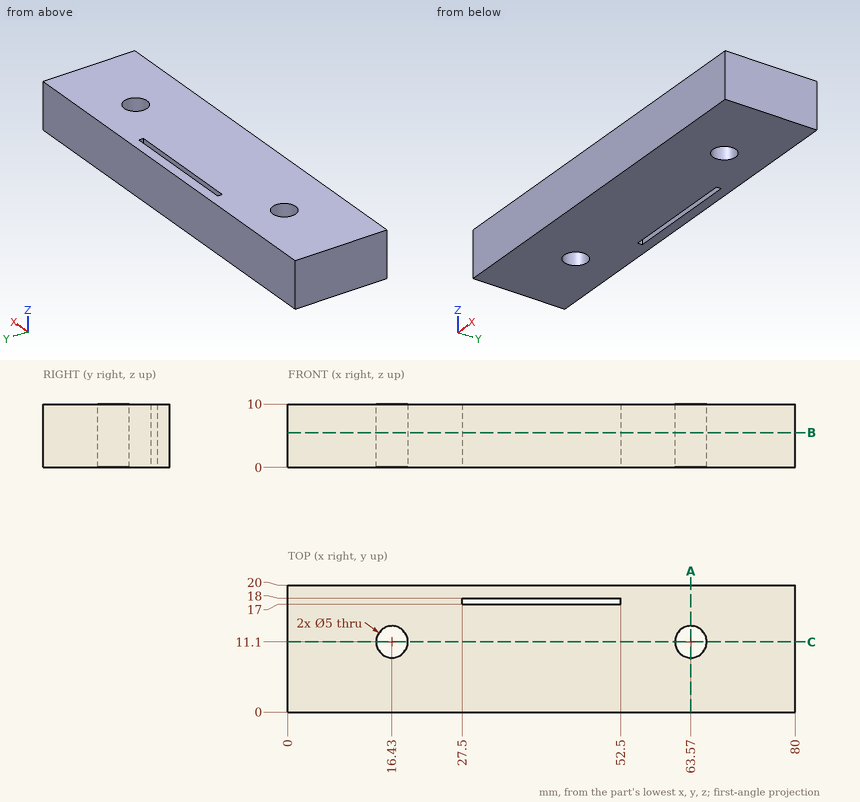
Source: three-view drawing plus pictorial views. Frame: mm from the lowest corner of the part. Give positions to 0.01 mm unless a question says otherwise; leave off trailing zeros. Order: outer loops, then holes, each group sorted by start corner. A loop starts at its lowest first (then second) coordinate and runs counter-clockwise, first axis right, second up. Notation, with made-up numbers: (-21, -11.5) -> (-8, -11.5) arc R27 ccw to (-8, 25.5) -> close; hole circle Ø8 at (11.25, 62). An arc over 180 degrees is marked (long way). Put each result on its own line as item: value.
Q1. Material intervals for L1, parallel to X at y = 11.25, z = 0.75; L2, parallel to Y at x = 63.57, z = 2.75; L3, parallel to X at y = 10, z = 8 (3 decimals), sorted ascending.
Here are the results:
L1: x = 0 to 13.93, 18.93 to 61.07, 66.07 to 80
L2: y = 0 to 8.6, 13.6 to 20
L3: x = 0 to 14.185, 18.675 to 61.325, 65.815 to 80
Q2. Section C-C, the plane y = 11.1. Return loops of the section in (x, z), then the cut area to 3 significant figures.
Here are the results:
outline: (0, 0) -> (13.93, 0) -> (13.93, 10) -> (0, 10) -> close; (18.93, 0) -> (61.07, 0) -> (61.07, 10) -> (18.93, 10) -> close; (66.07, 0) -> (80, 0) -> (80, 10) -> (66.07, 10) -> close
area: 700 mm^2
Q3. Section B-B, the plane z = 5.5. Return loops of the section in (x, y).
Here are the results:
outline: (0, 0) -> (80, 0) -> (80, 20) -> (0, 20) -> close; hole circle Ø5 at (16.43, 11.1); hole (27.5, 17) -> (52.5, 17) -> (52.5, 18) -> (27.5, 18) -> close; hole circle Ø5 at (63.57, 11.1)
Q4. Section A-A, the plane x = 63.57. Return loops of the section in (y, z).
Here are the results:
outline: (0, 0) -> (8.6, 0) -> (8.6, 10) -> (0, 10) -> close; (13.6, 0) -> (20, 0) -> (20, 10) -> (13.6, 10) -> close
